Can you work these out from the drawing? Everything is in mm from the part's minimum corner. Coordinates: 2 decimals unless noted, no trailing zeros. Loops run counter-clockwise (first coordinate to the right, second up) from the corner with the lowest first, then second, coordinate; pieces in that order, holes last. Notation, with made-up numbers: (44.5, -32) -> (83.5, -32) arc R29 cw to (83.5, 6) -> close; hole circle Ø11 at (-35.5, 17.5). An arc over 180 degrees is marked (long way). One line per question, with ' | ' between items.
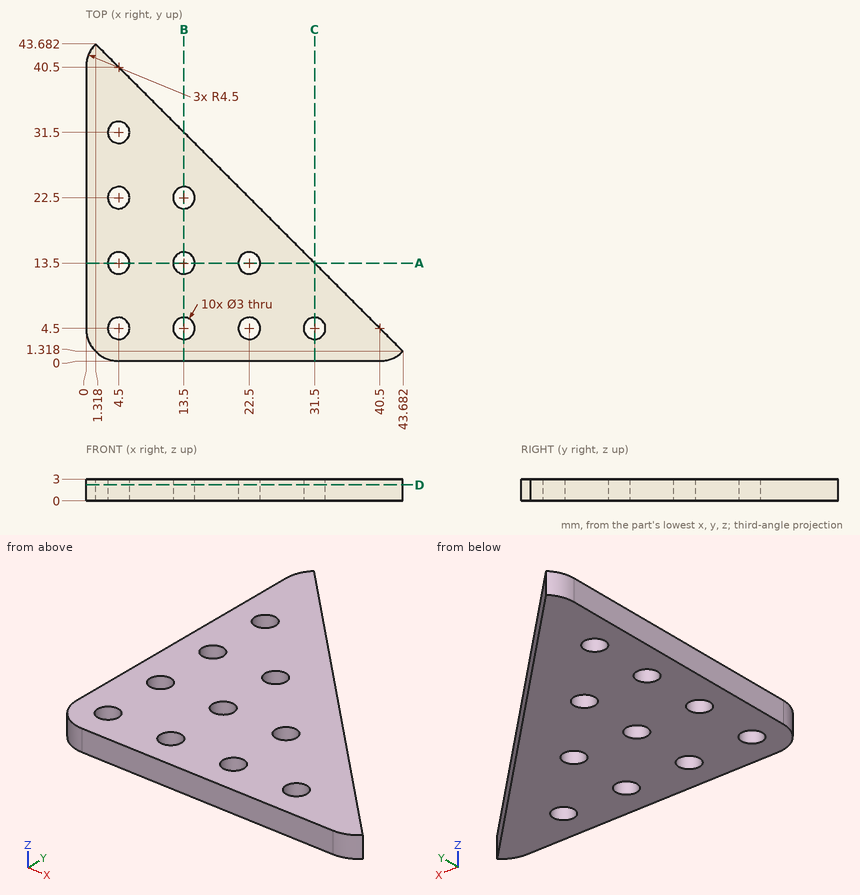
Q1. Please list where these lines run through material, in increasing order: L1, parallel to Y at x = 4.5, z = 1.55; L2, parallel to X at y = 5, z = 2.95; L3, parallel to Y at x = 13.5, z = 1.65. Write a range as [from, to].
Values follow:
L1: y = [0, 3], [6, 12], [15, 21], [24, 30], [33, 40.5] | L2: x = [0, 3.09], [5.91, 12.09], [14.91, 21.09], [23.91, 30.09], [32.91, 40] | L3: y = [0, 3], [6, 12], [15, 21], [24, 31.5]
Q2. Imagine slicing it at C-C on x = 31.5. Write out the boundary of the cut face in (y, z), plus the area to 3 significant figures.
Values follow:
outline: (0, 0) -> (3, 0) -> (3, 3) -> (0, 3) -> close; (6, 0) -> (13.5, 0) -> (13.5, 3) -> (6, 3) -> close | area: 31.5 mm2
Q3. Imagine slicing it at A-A on y = 13.5. Write out the boundary of the cut face in (x, z).
Values follow:
outline: (0, 0) -> (3, 0) -> (3, 3) -> (0, 3) -> close; (6, 0) -> (12, 0) -> (12, 3) -> (6, 3) -> close; (15, 0) -> (21, 0) -> (21, 3) -> (15, 3) -> close; (24, 0) -> (31.5, 0) -> (31.5, 3) -> (24, 3) -> close
Q4. For pin 1 (1 mm diameter, centred on x = 31, z = 1, fed in from +Y), with a flat end and sliding along its axis, tell me the tip position at first contact or that it passes through.
Values follow:
pin 1: stops at y = 14.5
Q5. Imagine slicing it at D-D on z = 2.2. Give the number of separate pieces and of enclosed holes in the cut face, plus the area to 3 significant figures.
Values follow:
separate pieces: 1 | enclosed holes: 10 | area: 933 mm2
